Check sheet for the modelled part. Datum: model origin and axes. Units: mm. A direction names the side the tool comes from. Give positions to 0.01 mm unless a question says otherwise; leave off trailing zeros. Loops run counter-clockwise (first coordinate to the right, second up) from the corner with the lowest first, then second, coordinate; pieces in that order, holes last. Notation, with made-up numbers: (-9, 71) - (-5, 71) arc R15 ccw to (-5, 82) - close; hole circle Ø7 at (-31, 36.5). An arc over 180 degrees is marked (long way). Answer in a Markdown table with one row per item. Add a question column.
(1) Sectioned sample at C-C on z = 117.5. Enter the section's corners in (x, y).
(2) Set-up check for faces 1 (the face through (9, -40.64, -10)), 2 (the face through (9.266, -109.284, 92.972)), 3 (the face through (9, -102, 0)), 4 (the face through (9, -183, 0)): record each of +Z, -Z, +X, -X, +Y, -Y from which the full face is reachable in a straight line by a thin tool's end or side.
(3) Thickness scan on L1, parallel to Y at x = 6.5, z = 152.5; L2, parallel to Y at x = 6.25, z = 226.5; L3, parallel to Z at x = 8.5, y = -124. Record the ranges inside material, lowest first.
(4) Sectioned sample at A-A on x = 11.25. Enter the section's corners in (y, z), then the cut area to 3 significant figures.
(5) Sectioned sample at B-B on y = -135.5. Enter the section's corners in (x, z), then the cut area to 3 significant figures.
(6) Draft check along Z on faces 5 (the face through (0, -80, 95)), 6 (the face through (9.27, -63.66, 198.2)), 7 (the face through (9, -143, -18.796)), 8 (the face through (9.266, -37.217, 228.097)). Enter one of: released by +Z, released by -Z, zero draft, split by the parting line, or undercut.
(7) Sectioned sample at D-D on z = 300. Enter the section's corners in (x, y), then the cut area to 3 significant figures.
(8) Go/stop test with flat-tipped pins: P1, Ø2, axis at x = 16.5, y = -100, coming from the +Z side (3 decimals); P2, Ø4, axis at x = 16, y = -24.5, coming from the +Z side; P3, Ø5.5, axis at x = 9, z = -7, coming from the -Y side. Record where each tip stops, or that it passes through.
from build123d import *

# Parameters (mm, degrees)
F0_W     = 40.64
F0_H     = 18.796
F1_DEPTH = 18.796


with BuildPart() as f1:
    # F0 (on Right) → F1 (new body)
    with BuildSketch(Plane.YZ):
        Polygon((-40.64, 0), (0, 0), (0, 337.82), (-36.037321, 270.250024), (-19.452615, 261.404847), (-55.485951, 193.842341), (-72.070657, 202.687518), (-108.103994, 135.125012), (-91.519288, 126.279835), (-127.552624, 58.717329), (-144.13733, 67.562506), (-180.170667, 0), (-162.56, 0), (-121.92, 0), (-101.6, 0), (-81.28, 0), align=None)
        Polygon((-36.037321, 270.250024), (0, 337.82), (0, 381), (-203.2, 0), (-180.170667, 0), (-144.13733, 67.562506), (-108.103994, 135.125012), (-72.070657, 202.687518), align=None)
        with Locations((-60.96, -9.398)):
            Rectangle(F0_W, F0_H)
        with Locations((-142.24, -9.398)):
            Rectangle(F0_W, F0_H)
    extrude(amount=F1_DEPTH)


solid = f1.part
Reply:
| question | item | result |
|---|---|---|
| 1 | outline | (0, -140.53) - (18.8, -140.53) - (18.8, -117.5) - (0, -117.5) - close; (0, -96.2) - (18.8, -96.2) - (18.8, 0) - (0, 0) - close |
| 2 | face 1 | -Z, +X, -X, +Y |
| 2 | face 2 | +X, -X |
| 2 | face 3 | -Z, +X, -X |
| 2 | face 4 | -Z, +X, -X, -Y |
| 3 | L1 | -121.87 to 0 |
| 3 | L2 | -82.4 to -59.37, -38.07 to 0 |
| 3 | L3 | -18.8 to 65.38, 105.32 to 148.5 |
| 4 | outline | (-203.2, 0) - (-162.56, 0) - (-162.56, -18.8) - (-121.92, -18.8) - (-121.92, 0) - (-81.28, 0) - (-81.28, -18.8) - (-40.64, -18.8) - (-40.64, 0) - (0, 0) - (0, 381) - close; hole (-144.14, 67.56) - (-127.55, 58.72) - (-91.52, 126.28) - (-108.1, 135.13) - close; hole (-72.07, 202.69) - (-55.49, 193.84) - (-19.45, 261.4) - (-36.04, 270.25) - close |
| 4 | area | 37,400 mm^2 |
| 5 | outline | (0, -18.8) - (18.8, -18.8) - (18.8, 62.96) - (0, 62.96) - close; (0, 83.76) - (18.8, 83.76) - (18.8, 126.94) - (0, 126.94) - close |
| 5 | area | 2,350 mm^2 |
| 6 | face 5 | zero draft |
| 6 | face 6 | undercut |
| 6 | face 7 | released by -Z |
| 6 | face 8 | undercut |
| 7 | outline | (0, -43.2) - (18.8, -43.2) - (18.8, 0) - (0, 0) - close |
| 7 | area | 812 mm^2 |
| 8 | P1 | z = 195.375 |
| 8 | P2 | z = 338.81 |
| 8 | P3 | y = -162.56 |
